Here's the drawing with two shaded views (mm, measured from the low corner). I have some questions. A direction names the side the tool comes from. Coordinates: 2 decimals unless noted, no trailing zeros. Order: outer loops, then holes, each group sorted by start corner. A loop starts at its lowest first (then second) coordinate and runs counter-clockwise, first axis right, second up. Notation, with made-up numbers: (-39.5, 48.25) -> (11.5, 48.25) arc R28 ccw to (11.5, 79.25) -> close; hole circle Ø11 at (-20.5, 29). An arc over 180 degrees is marked (long way). Answer as a JSON object with one key per item and string values. Group by question number.
(1) Which directions (+Z, -Z, +X, -X, +Y, -Y) give clear straight access to the entire face, cutting with the end or side of a thin tool? Please do the marked faces 1 and 2.
(2) For pin 1 (12 mm diameter, centred on x = 25, z = 40.5, fed in from +Y) (1 decimal); pin 2 (5 mm diameter, centred on x = 58, y = 61, fed in from -Z); pin 3 (1.5 mm diameter, centred on x = 77.5, y = 48.5, fed in from +Z); pin 4 (10 mm diameter, centred on x = 58.5, z = 32.5, fed in from +Y) (1 decimal), each with a flat end and sliding along its axis, tell me the tip position at first contact or that it passes through.
(3) I need wall thicknesses on line 1 (X direction, y = 31, z = 43.5); line 2 (Z direction, x = 12, y = 37); line 3 (Y direction, x = 46, z = 65.5). Which ranges of each line are inside material? Lowest first, please.
(4) I want a section at B-B, the plane z = 36. List the corners of the cut face in (x, y) for me, plus the area to 3 significant figures.
(5) I want a section at A-A, the plane z = 54. List the corners of the cut face in (x, y) for me, plus the area to 3 significant figures.
(6) If we mould it in two halves opening along X, with no side actions, what happens to the marked faces 3 and 4? For each: pulls with the +X half, pulls with the -X half, needs draft (parallel to the pull), parting line crosses it, or undercut.
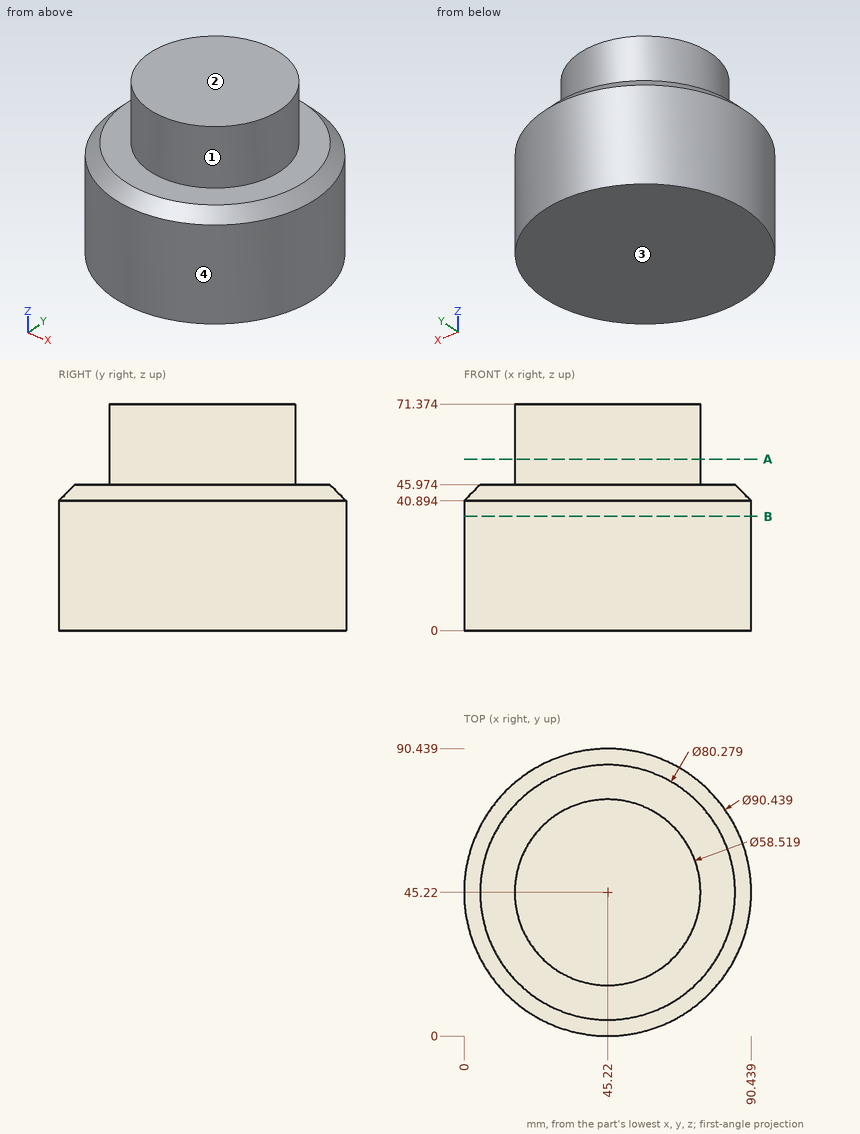
Computed values:
{
 "1": {"face 1": "+Z", "face 2": "+Z, +X, -X, +Y, -Y"},
 "2": {"pin 1": "stops at y = 88.1", "pin 2": "stops at z = 0", "pin 3": "stops at z = 45.97", "pin 4": "stops at y = 89.7"},
 "3": {"line 1": "x = 5.05 to 85.39", "line 2": "z = 0 to 45.97", "line 3": "y = 15.97 to 74.47"},
 "4": {"outline": "circle Ø90.44 at (45.22, 45.22)", "area": "6,420 mm2"},
 "5": {"outline": "circle Ø58.52 at (45.22, 45.22)", "area": "2,690 mm2"},
 "6": {"face 3": "needs draft", "face 4": "parting line crosses it"}
}
